Geometry: final body of the model. Coordinates: model frame, mm. Give positions to 0.01 mm unless a question says otherwise; leave off trailing zeros. Use CSV: the item, a comma, the result in double quotes.
```python
from build123d import *

# Parameters (mm, degrees)
RESSALTO_EXTRUS_O1_DEPTH = 300


with BuildPart() as part:
    # Esboço1 → Ressalto-extrusão1 (new body)
    with BuildSketch(Plane.XY):
        with BuildLine():
            Line((0, 0), (-113, 0))
            Line((-113, 0), (-113, 30))
            Line((-113, 30), (-111, 30))
            Line((-111, 30), (-111, 6))
            Line((-111, 6), (-107.3, 6))
            Line((-107.3, 6), (-106.5, 29))
            ThreePointArc((-106.5, 29), (-105.5, 30), (-104.5, 29))
            Line((-104.5, 29), (-104, 6))
            Line((-104, 6), (-100.3, 6))
            Line((-100.3, 6), (-99.5, 29))
            ThreePointArc((-99.5, 29), (-98.5, 30), (-97.5, 29))
            Line((-97.5, 29), (-97, 6))
            Line((-97, 6), (-93.3, 6))
            Line((-93.3, 6), (-92.5, 29))
            ThreePointArc((-92.5, 29), (-91.5, 30), (-90.5, 29))
            Line((-90.5, 29), (-90, 6))
            Line((-90, 6), (-86.3, 6))
            Line((-86.3, 6), (-85.5, 29))
            ThreePointArc((-85.5, 29), (-84.5, 30), (-83.5, 29))
            Line((-83.5, 29), (-83, 6))
            Line((-83, 6), (-79.3, 6))
            Line((-79.3, 6), (-78.5, 29))
            ThreePointArc((-78.5, 29), (-77.5, 30), (-76.5, 29))
            Line((-76.5, 29), (-76, 6))
            Line((-76, 6), (-72.3, 6))
            Line((-72.3, 6), (-71.5, 29))
            ThreePointArc((-71.5, 29), (-70.5, 30), (-69.5, 29))
            Line((-69.5, 29), (-69, 6))
            Line((-69, 6), (-65.3, 6))
            Line((-65.3, 6), (-64.5, 29))
            ThreePointArc((-64.5, 29), (-63.5, 30), (-62.5, 29))
            Line((-62.5, 29), (-62, 6))
            Line((-62, 6), (-58.3, 6))
            Line((-58.3, 6), (-57.5, 29))
            ThreePointArc((-57.5, 29), (-56.5, 30), (-55.5, 29))
            Line((-55.5, 29), (-54.7, 6))
            Line((-54.7, 6), (-51, 6))
            Line((-51, 6), (-50.5, 29))
            ThreePointArc((-50.5, 29), (-49.5, 30), (-48.5, 29))
            Line((-48.5, 29), (-47.7, 6))
            Line((-47.7, 6), (-44, 6))
            Line((-44, 6), (-43.5, 29))
            ThreePointArc((-43.5, 29), (-42.5, 30), (-41.5, 29))
            Line((-41.5, 29), (-40.7, 6))
            Line((-40.7, 6), (-37, 6))
            Line((-37, 6), (-36.5, 29))
            ThreePointArc((-36.5, 29), (-35.5, 30), (-34.5, 29))
            Line((-34.5, 29), (-33.7, 6))
            Line((-33.7, 6), (-30, 6))
            Line((-30, 6), (-29.5, 29))
            ThreePointArc((-29.5, 29), (-28.5, 30), (-27.5, 29))
            Line((-27.5, 29), (-26.7, 6))
            Line((-26.7, 6), (-23, 6))
            Line((-23, 6), (-22.5, 29))
            ThreePointArc((-22.5, 29), (-21.5, 30), (-20.5, 29))
            Line((-20.5, 29), (-19.7, 6))
            Line((-19.7, 6), (-16, 6))
            Line((-16, 6), (-15.5, 29))
            ThreePointArc((-15.5, 29), (-14.5, 30), (-13.5, 29))
            Line((-13.5, 29), (-12.7, 6))
            Line((-12.7, 6), (-9, 6))
            Line((-9, 6), (-8.5, 29))
            ThreePointArc((-8.5, 29), (-7.5, 30), (-6.5, 29))
            Line((-6.5, 29), (-5.7, 6))
            Line((-5.7, 6), (-2, 6))
            Line((-2, 6), (-2, 30))
            Line((-2, 30), (0, 30))
            Line((0, 30), (0, 0))
        make_face()
    extrude(amount=RESSALTO_EXTRUS_O1_DEPTH)


solid = part.part
```
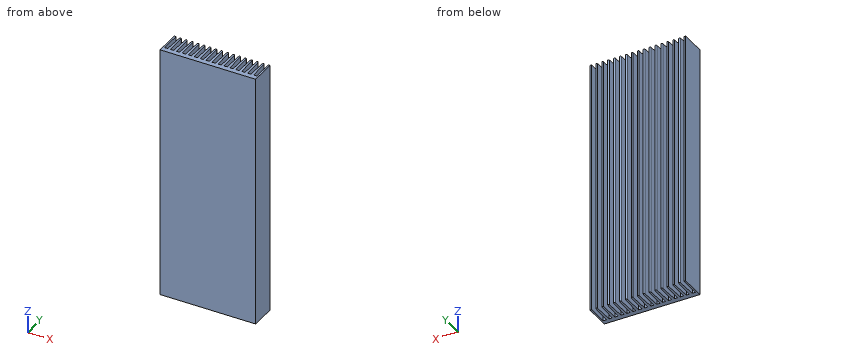
1. Line query: line 1 (Y direction, x = -18, z = 254.5); line 2 (Y direction, x = -106, z = 23.5). Output: solid intervals per line, ascending.
Answer:
line 1,"0 to 6"
line 2,"0 to 29.87"
2. Pin query (flat end, axial travel): pin 1 Ø3 at (x, z) = (-81, 196) entering from +Y; pin 2 Ø6 at (x, y) = (-71, 19.5) entering from -Z; pin 3 Ø1.5 at (x, z) = (-58, 190.5) entering from +Y. Return the tip coordinate at first contact, or that it passes through.
Answer:
pin 1,"y = 6"
pin 2,"z = 0"
pin 3,"y = 29.66"
3. Section A-A, the plane y = 20. Give the number of separate pieces and of enclosed holes in the cut face, plus the area to 3 significant figures.
Answer:
separate pieces,"17"
enclosed holes,"0"
area,"12,500 mm2"
